from build123d import *

# Parameters (mm, degrees)
SKETCH1_W                                          = 44
SKETCH1_H                                          = 15.3
BOSS_EXTRUDE1_DEPTH                                = 2.5
CBORE_FOR_M2_5_PAN_HEAD_MACHINE_SCREW1_D           = 2.7
CBORE_FOR_M2_5_PAN_HEAD_MACHINE_SCREW1_CBORE_D     = 6
CBORE_FOR_M2_5_PAN_HEAD_MACHINE_SCREW1_CBORE_DEPTH = 1
CUT_EXTRUDE1_DEPTH                                 = 1
FILLET1_R                                          = 1
FILLET2_R                                          = 0.25


with BuildPart() as part:
    # Sketch1 → Boss-Extrude1 (new body)
    with BuildSketch(Plane(origin=(0, 0, 0), x_dir=(0, 0, -1), z_dir=(1, 0, 0))):
        Rectangle(SKETCH1_W, SKETCH1_H)
    extrude(amount=BOSS_EXTRUDE1_DEPTH)

    # CBORE for M2.5 Pan Head Machine Screw1 (through all)
    with Locations(Plane(origin=(2.5, 0, 0), x_dir=(0, 0, -1), z_dir=(1, 0, 0))):
        with Locations((-19.5, 5), (18.125, 5)):
            CounterBoreHole(CBORE_FOR_M2_5_PAN_HEAD_MACHINE_SCREW1_D / 2, CBORE_FOR_M2_5_PAN_HEAD_MACHINE_SCREW1_CBORE_D / 2, CBORE_FOR_M2_5_PAN_HEAD_MACHINE_SCREW1_CBORE_DEPTH)

    # Sketch5 → Cut-Extrude1 (cut)
    with BuildSketch(Plane(origin=(2.5, 0, 0), x_dir=(0, 0, -1), z_dir=(1, 0, 0))):
        with BuildLine():
            ThreePointArc((-20.906236111, 7.65), (-21.515075982, 7.222491571), (-22, 6.658312395))
            Line((-22, 6.658312395), (-22, 7.65))
            Line((-22, 7.65), (-20.906236111, 7.65))
        make_face()
    extrude(amount=-CUT_EXTRUDE1_DEPTH, mode=Mode.SUBTRACT)

    # Fillet1
    fillet1_edges = [part.edges().sort_by_distance(p)[0] for p in [
        (2, 7.65, -16.718763889),
        (2, 7.65, 18.093763889),
        (2, 3.341687605, 22),
        (0.75, 7.65, 22),
        (1.25, -7.65, -22),
        (1.25, -7.65, 22),
        (1.25, 7.65, -22),
    ]]
    fillet(fillet1_edges, radius=FILLET1_R)

    # Fillet2
    fillet2_edges = [part.edges().sort_by_distance(p)[0] for p in [
        (2, 7.65, -19.531236111),
    ]]
    fillet(fillet2_edges, radius=FILLET2_R)


solid = part.part
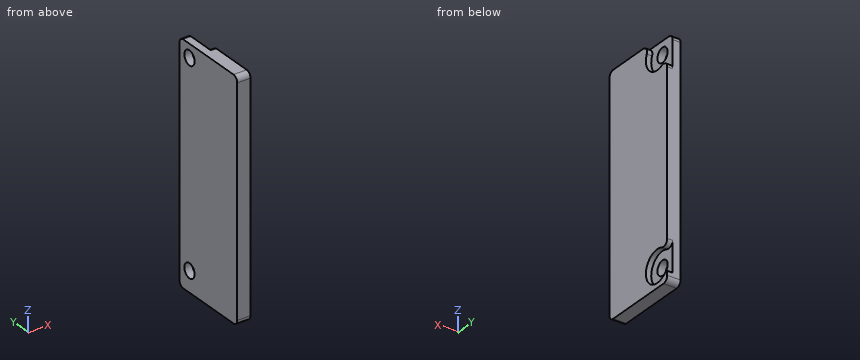
Part model, mm, in its own coordinate system. Give positions to 0.01 mm unless a question says otherwise; leave off trailing zeros. Loops run counter-clockwise (first coordinate to the right, second up) from the corner with the lowest first, then second, coordinate; pieces in that order, holes last.
(1) Band-saw the part on A-A (z = 19.5). Write the cut outline in (x, y).
Return value:
outline: (0, -7.65) - (2.5, -7.65) - (2.5, 2) - (1.5, 2) - (1.5, 3.65) - (0, 3.65) - close; (0, 6.35) - (1.5, 6.35) - (1.5, 7.65) - (0, 7.65) - close
(2) Band-saw the part on D-D (z = -17.5). Write the cut outline in (x, y).
Return value:
outline: (0, -7.65) - (2.5, -7.65) - (2.5, 2.07) - (1.5, 2.07) - (1.5, 3.8) - (0, 3.8) - close; (0, 6.2) - (1.5, 6.2) - (1.5, 7.65) - (0, 7.65) - close
(3) Drill centre lines: line 1 along Z through (x, y) = (1.3, 5.75); line 2 along Z through (x, y) = (2.05, 5) (3 decimals); line 3 along Z through (x, y) = (1.7, 5.5). Where is each one in solid material? Low to high.
Return value:
line 1: z = -22 to -19.25, -17 to 18.38, 20.62 to 22
line 2: z = -22 to -21.125, -15.125 to 16.5
line 3: z = -22 to -21.08, -15.17 to 16.54
(4) Band-saw the part on C-C (x = 0.85). Write the cut outline in (y, z) (3 decimals).
Return value:
outline: (-7.65, -21) arc R1 ccw to (-6.65, -22) - (6.65, -22) arc R1 ccw to (7.65, -21) - (7.65, 21) arc R1 ccw to (6.65, 22) - (-6.65, 22) arc R1 ccw to (-7.65, 21) - close; hole circle Ø2.7 at (5, -18.125); hole circle Ø2.7 at (5, 19.5)
(5) Band-saw the part on B-B (y = 5). Write the cut outline in (x, z) (3 decimals).
Return value:
outline: (0, -22) - (2.5, -22) - (2.5, -21.125) - (1.5, -21.125) - (1.5, -19.475) - (0, -19.475) - close; (0, -16.775) - (1.5, -16.775) - (1.5, -15.125) - (2.5, -15.125) - (2.5, 16.5) - (1.5, 16.5) - (1.5, 18.15) - (0, 18.15) - close; (0, 20.85) - (1.5, 20.85) - (1.5, 22) - (0, 22) - close
(6) Pin check, flat tips, straight feed: pin 1 (2.5 mm diameter, centred on y = 5, z = 19.5, fed in from -X); pin 2 (5 mm diameter, centred on y = 5.5, z = 20, fed in from +X). Stop position of each tip, or through.
Return value:
pin 1: passes through
pin 2: stops at x = 1.5
